Geometry check sheet. Reference: drawing and pictorial views, mm from the part's lowest x, y, z. Round coordinates to 2 decimals unless told otherwise and drop trailing zeros. Loops run counter-clockwise (first coordinate to the right, second up) from the corner with the lowest first, then second, coordinate; pieces in that order, holes last. Notation, with made-up numbers: (61, 50) - (114, 50) arc R25 cw to (114, 68) - close; hole circle Ø8 at (18.25, -2). An arc over 180 degrees is marked (long way). Answer in a Markdown table with one row per item. Add a question column.
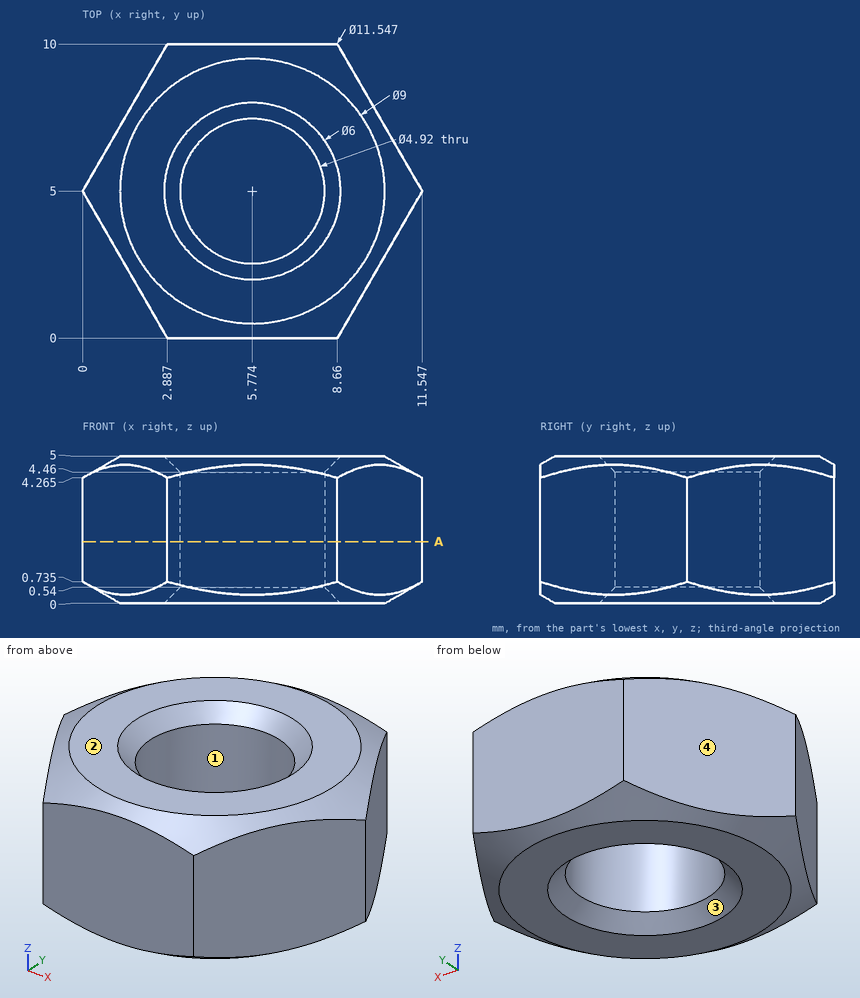
Q1. Release check for a two-part mould opening along X. For the marked faces 1, 2, 3 and 4 record: +X half, -X half, draft (parallel to the pull), parting line (faces both ways), or undercut.
Q2. Scan lines: line 1 (Y direction, x = 5, z = 1.55) (1 decimal); line 2 (Y direction, x = 7.75, z = 0.9) (1 decimal); line 3 (X direction, y = 2, z = 0.65) (1 decimal). Record each from-to range of solid material in increasing order. Write a range as from..to.
Q3. Depth check by flat-ended pin: P1, Ø1.5, axis at y = 6.5, z = 0.5, coming from the +X side (1 decimal); P2, Ø3, axis at x = 1.5, z = 1, coming from the -Y side; P3, Ø2, axis at y = 7.5, z = 4.5, coming from the -X side (1 decimal). Enter the tip coordinate at first touch or a pass-through.
Q4. Cross-section at A-A, the plane z = 2.1. Enter the section's corners in (x, y).
Check sheet entries:
| question | item | result |
|---|---|---|
| 1 | face 1 | undercut |
| 1 | face 2 | draft |
| 1 | face 3 | undercut |
| 1 | face 4 | -X half |
| 2 | line 1 | 0..2.7, 7.3..10 |
| 2 | line 2 | 0..3.5, 6.5..10 |
| 2 | line 3 | 1.7..9.8 |
| 3 | P1 | x = 11.1 |
| 3 | P2 | y = 0 |
| 3 | P3 | x = 0.9 |
| 4 | outline | (0, 5) - (2.89, 0) - (8.66, 0) - (11.55, 5) - (8.66, 10) - (2.89, 10) - close; hole circle Ø4.92 at (5.77, 5) |
